Could you check a few things on this drawing? It's one solid part, dimensions in mm from its lowest x, y, z. Round coordinates to 2 decimals unless told otherwise and drop trailing zeros. Order: outer loops, then holes, each group sorted by start corner. A loop starts at its lowest first (then second) coordinate and runs counter-clockwise, first axis right, second up. Notation, with made-up numbers: (-28.5, 16) - (8.5, 16) arc R37 cw to (8.5, 52) - close; hole circle Ø3 at (-39.5, -34.5). An arc over 180 degrees is marked (long way). Use one line per item in the form item = value.
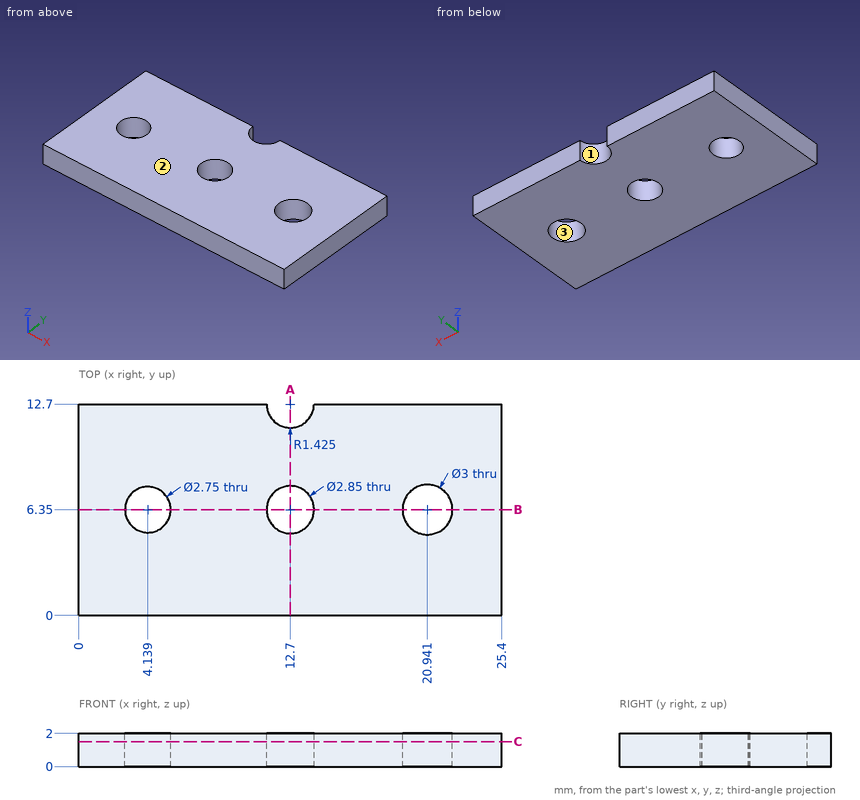
Item 1: Will this pin go through, and if not, where does the flat tip stop? P1, Ø6, axis at x = 17.5, y = 8, coming from the -Z side.
Found:
P1 = 0
Item 2: Imagine slicing it at B-B on y = 6.35. Please give me the cut outline in (x, z) (3 decimals), plus the area to 3 significant figures.
Found:
outline = (0, 0) - (2.764, 0) - (2.764, 2) - (0, 2) - close; (5.514, 0) - (11.275, 0) - (11.275, 2) - (5.514, 2) - close; (14.125, 0) - (19.441, 0) - (19.441, 2) - (14.125, 2) - close; (22.441, 0) - (25.4, 0) - (25.4, 2) - (22.441, 2) - close
area = 33.6 mm2
Item 3: If we mould it in two halves opening along X, with no side actions, what happens to the marked faces 1, 2 and 3? For each: released by +X, released by -X, zero draft, split by the parting line, or undercut.
Found:
face_1 = undercut
face_2 = zero draft
face_3 = undercut
Item 4: Imagine slicing it at A-A on x = 12.7. Please give me the cut outline in (y, z) (3 decimals).
Found:
outline = (0, 0) - (4.925, 0) - (4.925, 2) - (0, 2) - close; (7.775, 0) - (11.275, 0) - (11.275, 2) - (7.775, 2) - close
Item 5: I need wall thicknesses on L1, parallel to X at y = 6.35, z = 1.05 (3 decimals); L2, parallel to Y at x = 12.7, z = 1.35 (3 decimals); L3, parallel to X at y = 11.75, z = 1.4. Which ranges of each line are inside material? Lowest first, please.
Found:
L1 = 0 to 2.764, 5.514 to 11.275, 14.125 to 19.441, 22.441 to 25.4
L2 = 0 to 4.925, 7.775 to 11.275
L3 = 0 to 11.64, 13.76 to 25.4
Item 6: Imagine slicing it at C-C on z = 1.5. Please give me the cut outline in (x, y) (3 decimals).
Found:
outline = (0, 0) - (25.4, 0) - (25.4, 12.7) - (14.125, 12.7) arc R1.425 cw to (11.275, 12.7) - (0, 12.7) - close; hole circle Ø2.75 at (4.139, 6.35); hole circle Ø2.85 at (12.7, 6.35); hole circle Ø3 at (20.941, 6.35)
